Could you check a few things on this model? Use its own coordinates, in mm. A direction names the side the tool comes from. Give positions to 0.01 mm unless a question says otherwise; leave off trailing zeros. Order: outer loops, then holes, each group sorted by start corner. A loop starts at its lowest first (then second) coordinate and runs counter-clockwise, first axis right, second up. Notation, with made-up numbers: (78, 44) -> (98, 44) arc R27 cw to (98, 66) -> close; hole circle Ø7 at (30, 35). An arc over 180 degrees is marked (long way). Use one line per item in the form item = value. Start each with the question number.
Autodesk Inventor part; units mm, degrees
ref_plane "YZ Plane" through (0, 0, 0) normal (1, 0, 0) x (0, 1, 0)
ref_plane "XZ Plane" through (0, 0, 0) normal (0, 1, 0) x (-1, 0, 0)
ref_plane "XY Plane" through (0, 0, 0) normal (0, 0, 1) x (1, 0, 0)
ref_plane "Plano de trabajo1" through (19.2, 96.5, -0.8) normal (0, 1, 0) x (0, 0, -1)
sketch "Boceto1" plane through (19.2, 96.5, -0.8) normal (0, 1, 0) x (0, 0, -1)
  line L0 (-0.8, -18.4634) -> (-0.8, 18.4634)
  line L1 (-6.9748, 20) -> (-6.9748, -22)
  line L2 (-6.9748, -22) -> (21.3095, -50.2842)
  line L3 (-6.1748, 20) -> (283.8252, 20)
  line L4 (16.3598, -55.234) -> (-13.9748, -24.8995)
  line L5 (-13.9748, -24.8995) -> (-13.9748, 20)
  line L6 (21.3095, -50.2842) -> (16.3598, -55.234)
  line L7 (-6.9748, 20) -> (-13.9748, 20)
  point P0 (-0.8, 19.2)
  point P1 (-0.8, 18.4634)
  dimension "d0" = 135
  dimension "d1" = 42
  dimension "d2" = 40
  dimension "d3" = 7
extrude "Extrusión1" add sketch "Boceto1" against normal blind 40
chamfer "Chaflán1" distance 4 angle 45 1 edges at (69.4842, 76.5, -22.1095)
chamfer "Chaflán2" distance 4 angle 45 3 edges at (-0.8, 76.5, 13.1748) (21.6497, 96.5, 13.1748) (21.6497, 56.5, 13.1748)
sketch "Boceto2" plane through (3.2, 92.5, 13.1748) normal (0, 0, 1) x (1, 0, 0)
  circle A0 centre (6, -6) radius 2.5
  circle A1 centre (26, -5.9999) radius 2.6
  circle A2 centre (6, -26) radius 2.5
  point P0 (-3.2, -92.5)
hole "Agujero1" at (29.2, 86.5001, 13.1748) at (9.2, 66.5, 13.1748) direction (0, 0, -1) diameter 5.5 end through all counterbore diameter 10 counterbore depth 5.5
sketch "Boceto3" plane through (74.434, 56.5, -17.1598) normal (0.7071, 0, 0.7071) x (0.7071, 0, -0.7071)
  line L0 (114.1005, 77) -> (-42.8995, 77)
  line L1 (-42.8995, 77) -> (-42.8995, 0)
  line L2 (-42.8995, 0) -> (114.1005, 0)
  line L3 (114.1005, 0) -> (114.1005, 77)
  line L4 (-42.8995, 36) -> (-42.8995, 4)
  line L5 (0, 0) -> (-37.2426, 0)
  point P0 (-64.7666, -56.5)
  dimension "d19" = 157
  dimension "d20" = 77
extrude "Extrusión2" [suppressed]
equation "\"d17\" = Grosor"
equation "\"Profundidad_desahogo_plegado\" = 0.5 * Grosor"
properties part number "SoporteKlipperScreen"
(1) Imagine slicing it at C-C (x = 18). Write out the boundary of the cut face in (y, z), plus the area to 3 significant figures.
(2) Imagine slicing it at A-A (y = 66.5). Write out the boundary of the cut face in (x, z), plus the area to 3 significant figures.
(3) I'm going to push flat-ended pins straight in: pin 1 Ø8 at (y, z) = (77, -3) entering from +X; pin 2 Ø6.5 at (x, y) = (9.2, 66.5) entering from -Z; pin 3 Ø6 at (y, z) = (89.5, -10) entering from -X; pin 4 Ø6 at (x, z) = (54.5, 8.5) entering from +Y. Where does each tip first touch, or does it pass through?
(4) We'd pull the mould along X, two halves only. Please class faces 1 (the flat face through (53.75, 76.78, -6.375)), 2 (the flat face through (23.307, 58.528, 11.203)), 3 (the flat face through (31, 84, 7.675)): pulls with the +X half, pulls with the -X half, needs draft (parallel to the pull), parting line crosses it, or undercut.
(5) Which directions (+Z, -Z, +X, -X, +Y, -Y) give clear straight access to the entire face, cutting with the end or side of a thin tool? Please do faces 4 (the flat face through (23.307, 94.472, 11.203)), 5 (the flat face through (20, 77, 6.175)), 6 (the flat face through (11, 64, 7.675)).
(6) Please list where these lines run through material, in increasing order: probe 1 along Y at (x, z) = (29.2, 7.4); probe 2 along Y at (x, z) = (29, 9); probe 3 along Z at (x, y) = (40, 73).
(7) Imagine slicing it at D-D (y = 77). Write out the boundary of the cut face in (x, z), plus the area to 3 significant figures.
(8) Imagine slicing it at B-B (x = 9.2). Write out the boundary of the cut face in (y, z), plus the area to 3 significant figures.
Calculated:
q1.outline = (56.5, 6.17) -> (96.5, 6.17) -> (96.5, 9.17) -> (92.5, 13.17) -> (60.5, 13.17) -> (56.5, 9.17) -> close
q1.area = 264 mm2
q2.outline = (-0.8, 6.17) -> (6.45, 6.17) -> (6.45, 7.67) -> (4.2, 7.67) -> (4.2, 13.17) -> (3.2, 13.17) -> (-0.8, 9.17) -> close; (11.95, 6.17) -> (41.2, 6.17) -> (66.66, -19.28) -> (72.31, -19.28) -> (74.43, -17.16) -> (44.1, 13.17) -> (14.2, 13.17) -> (14.2, 7.67) -> (11.95, 7.67) -> close
q2.area = 515 mm2
q3.pin_1 = 64.27
q3.pin_2 = 6.17
q3.pin_3 = 54.37
q3.pin_4 = through
q4.face_1 = pulls with the -X half
q4.face_2 = needs draft
q4.face_3 = undercut
q5.face_4 = +Z, +X, -X, +Y
q5.face_5 = -Z, -X, +Y, -Y
q5.face_6 = +Z
q6.probe_1 = 56.5 to 83.75, 89.25 to 96.5
q6.probe_2 = 56.5 to 81.5, 91.5 to 96.5
q6.probe_3 = 6.17 to 13.17
q7.outline = (-0.8, 6.17) -> (41.2, 6.17) -> (66.66, -19.28) -> (72.31, -19.28) -> (74.43, -17.16) -> (44.1, 13.17) -> (3.2, 13.17) -> (-0.8, 9.17) -> close
q7.area = 578 mm2
q8.outline = (56.5, 6.17) -> (63.75, 6.17) -> (63.75, 7.67) -> (61.5, 7.67) -> (61.5, 13.17) -> (60.5, 13.17) -> (56.5, 9.17) -> close; (69.25, 6.17) -> (96.5, 6.17) -> (96.5, 9.17) -> (92.5, 13.17) -> (71.5, 13.17) -> (71.5, 7.67) -> (69.25, 7.67) -> close
q8.area = 201 mm2
